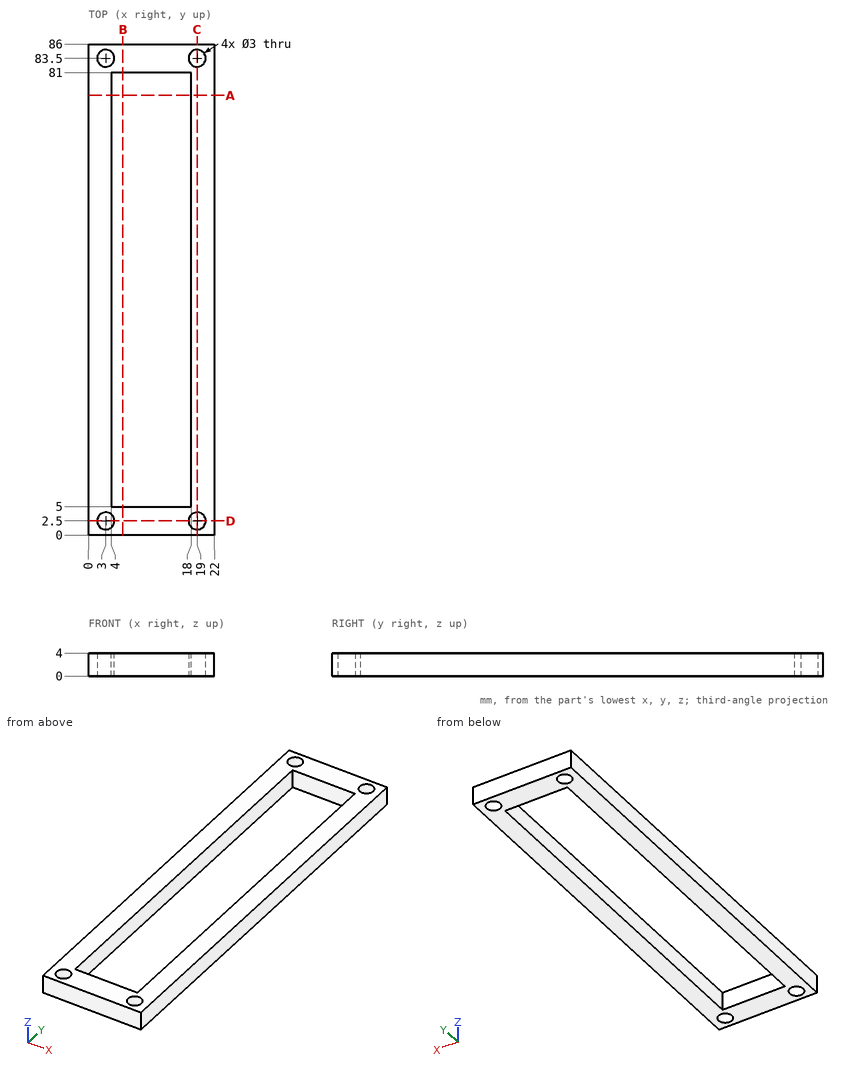
Design review of the part shown in the three views and the two pictorial views. Dimensions are in mm from the part's minimum x, y and z. Give positions to 0.01 mm unless a question says otherwise; leave off trailing zeros. Order: outer loops, then holes, each group sorted by start corner. A loop starts at its lowest first (then second) coordinate and runs counter-clockwise, first axis right, second up. Notation, with made-up numbers: (3.25, 44) -> (35.25, 44) arc R26 ccw to (35.25, 74) -> close; hole circle Ø2 at (16.5, 23). An arc over 180 degrees is marked (long way). Write each question's results on one line, items separated by ' | '. Start each with the question number.
Q1. Add section B-B on x = 6. Give the boundary of the cut face in (y, z), and give its area (3 significant figures).
Q2. Add section A-A on y = 77. Give the boundary of the cut face in (x, z), and give its area (3 significant figures).
Q3. Add section D-D on y = 2.5. Give the boundary of the cut face in (x, z).
Q4. Wall thickness on L1, parallel to Y at x = 19, z = 1.8; L2, parallel to X at y = 16.5, z = 2.4; L3, parallel to Y at x = 10.75, z = 3.75: over which ranges is each line inside the solid? List them lowest first. Write a range as from..to.
Q5. Add section C-C on x = 19. Give the boundary of the cut face in (y, z), and give its area (3 significant figures).
Q6. For pin 1 (8 mm diameter, centred on x = 19.5, y = 56.5, fed in from -Z); pin 2 (2.5 mm diameter, centred on x = 3, y = 83.5, fed in from +Z), all flat-tipped, find the tip position at first contact; note any pin that passes through.
Found:
1) outline: (0, 0) -> (5, 0) -> (5, 4) -> (0, 4) -> close; (81, 0) -> (86, 0) -> (86, 4) -> (81, 4) -> close | area: 40.0 mm2
2) outline: (0, 0) -> (4, 0) -> (4, 4) -> (0, 4) -> close; (18, 0) -> (22, 0) -> (22, 4) -> (18, 4) -> close | area: 32.0 mm2
3) outline: (0, 0) -> (1.5, 0) -> (1.5, 4) -> (0, 4) -> close; (4.5, 0) -> (17.5, 0) -> (17.5, 4) -> (4.5, 4) -> close; (20.5, 0) -> (22, 0) -> (22, 4) -> (20.5, 4) -> close
4) L1: y = 0..1, 4..82, 85..86 | L2: x = 0..4, 18..22 | L3: y = 0..5, 81..86
5) outline: (0, 0) -> (1, 0) -> (1, 4) -> (0, 4) -> close; (4, 0) -> (82, 0) -> (82, 4) -> (4, 4) -> close; (85, 0) -> (86, 0) -> (86, 4) -> (85, 4) -> close | area: 320 mm2
6) pin 1: stops at z = 0 | pin 2: passes through
